Drawing for the job (mm, zero at the part's lowest x, y, z). Give positions to 0.01 mm unless a question says otherwise; leave off trailing zeros. Order: outer loops, then holes, each group sorted by start corner. A loop starts at its lowest first (then second) coordinate and runs counter-clockwise, first axis right, second up. Notation, with made-up numbers: (3.25, -6.75) - (11.25, -6.75) arc R11 ccw to (11.25, 10.25) - close; hole circle Ø4 at (11, 15). An arc over 180 degrees is marked (long way). One line per item, written item: value.
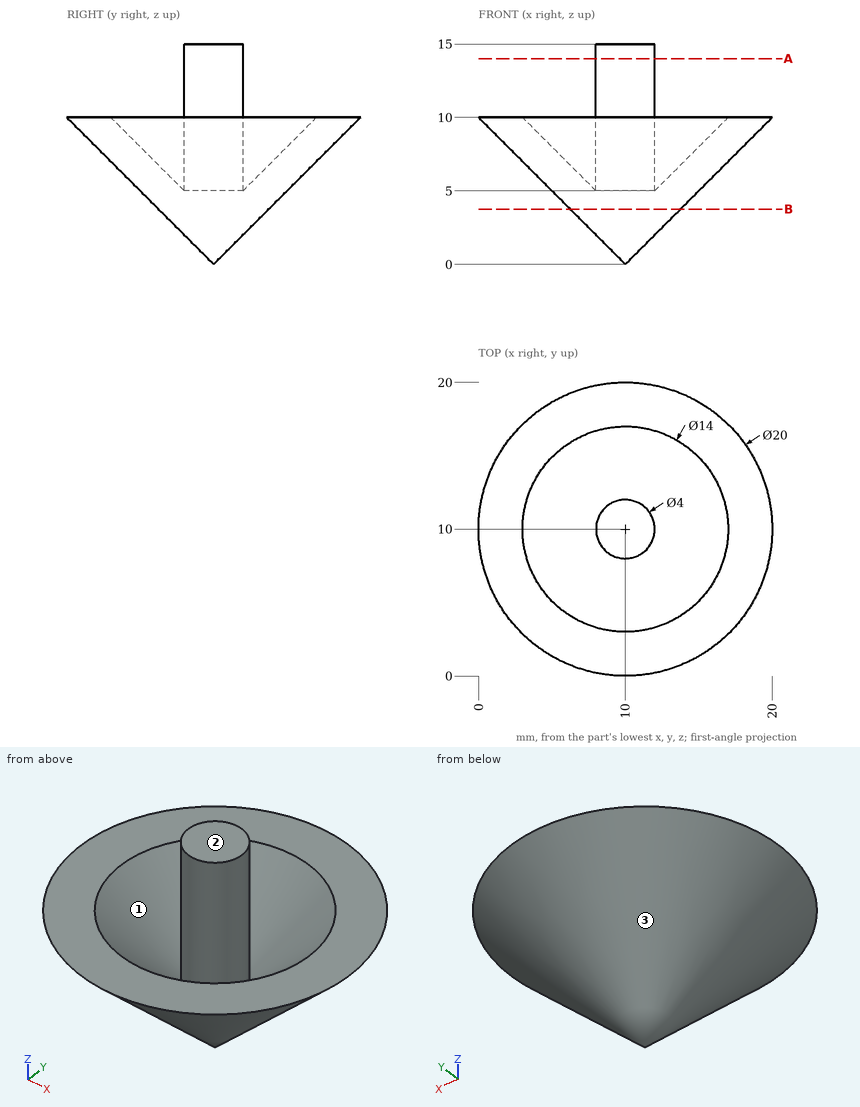
1) Cut at A-A, the plane z = 14. Give the cut face in (x, y), then the cut area to 3 significant figures.
Outcome:
outline: circle Ø4 at (10, 10)
area: 12.6 mm^2
2) Mould opens along Y. For the marked faces 1, 2 and 3 say: released by +Y, released by -Y, zero draft, split by the parting line, or undercut.
Outcome:
face 1: undercut
face 2: zero draft
face 3: split by the parting line
3) Drill centre lines: line 1 along Y through (x, z) = (15.25, 7.25); line 2 along Y through (x, z) = (13.25, 8.25); line 3 along Z through (x, y) = (10, 3.5). Where is each one in solid material? Low to high. Write a range as from..to.
Outcome:
line 1: y = 5..15
line 2: y = 2.42..5.88, 14.12..17.58
line 3: z = 6.5..9.5
4) Pin check, flat tips, straight feed: pin 1 (6 mm diameter, centred on x = 12, y = 10.5, fed in from +Z); pin 2 (4 mm diameter, centred on x = 5.5, z = 8, fed in from +Y); pin 3 (8 mm diameter, centred on x = 2.5, y = 13.5, fed in from +Z); pin 4 (1 mm diameter, centred on x = 12.5, z = 7.5, fed in from +Y). Stop position of each tip, or through.
Outcome:
pin 1: stops at z = 15
pin 2: stops at y = 19.11
pin 3: stops at z = 10
pin 4: stops at y = 17.62
5) Cut at B-B, the plane z = 3.75. Give the cut face in (x, y), then the cut area to 3 significant figures.
Outcome:
outline: circle Ø7.5 at (10, 10)
area: 44.2 mm^2
